Geometry check sheet. Reference: the model listing, model coordinates, mm. Give positions to 0.01 mm unless a question says otherwise; leave off trailing zeros. Loops run counter-clockwise (first coordinate to the right, second up) from the corner with the lowest first, then second, coordinate; pieces in that order, holes last. Notation, with made-up numbers: (50.5, 62.5) - (83.5, 62.5) arc R12 ccw to (83.5, 85.5) - close; hole circle Ø4 at (-33.5, 39). An arc over 180 degrees is marked (long way). Use a Markdown table: item, result. Add a question column.
1. Material ranges on L1, parallel to Y at x = -18, z = 6.25; L2, parallel to Z at x = -5, y = -38; L3, parallel to X at y = 27.5, z = 7, recorded low to high.
2. Cross-section at A-A on x = -6. Enter the section's corners in (y, z), and give its area (3 significant figures).
3. Depth check by flat-ended pin: P1, Ø0.8, axis at y = 30.5, z = 9.5, coming from the +X side; P2, Ø1.6, axis at x = -41, y = 10, coming from the +Z side. Enter the tip coordinate at first touch or a pass-through.
4. Cross-section at B-B on y = -40. Enter the section's corners in (x, z), and give its area (3 significant figures).
from build123d import *

# Parameters (mm, degrees)
F1_DEPTH = 132
F4_T     = -2


with BuildPart() as f1:
    # F0 (on Front) → F1 (new body)
    with BuildSketch(Plane.XZ):
        Polygon((-39.8409090909, -5.0908953616), (27.1590909091, -5.0908953616), (30.1590909091, -5.0908953616), (30.1590909091, -0.0908953616), (29.1590909091, 0.9091046384), (27.1590909091, 0.9091046384), (27.1590909091, 1.9091046384), (-39.8410601137, 1.909104627), (-39.8409090909, 0.9091046384), (-41.8409090909, 0.9088025928), (-42.8409090909, -0.0908953616), (-42.8409090909, -5.0908953616), align=None)
    extrude(amount=F1_DEPTH)


with BuildPart() as f1_1:
    # F2: moved
    add(f1.part.moved(Location((0, 0, 8))))


with BuildPart() as f1_2:
    # F3: moved
    add(f1_1.part.moved(Location((0, 70, 0))))

    # F4 (hollow: no face is removed)
    offset(amount=F4_T, kind=Kind.INTERSECTION, mode=Mode.SUBTRACT)


solid = f1_2.part
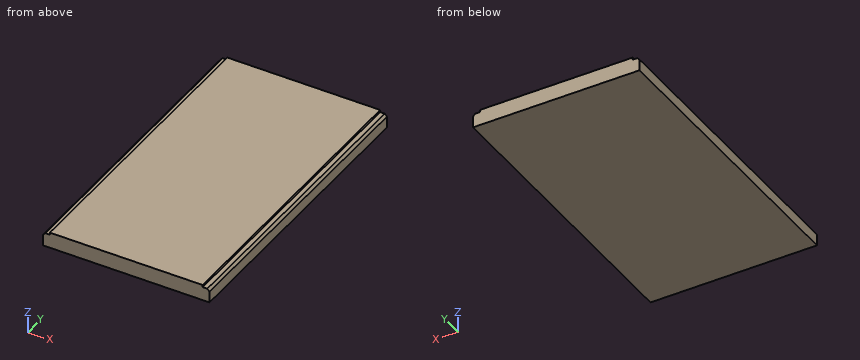
Values found:
| question | item | result |
|---|---|---|
| 1 | L1 | y = -62 to -60, 68 to 70 |
| 1 | L2 | z = 2.91 to 4.91, 7.91 to 9.91 |
| 1 | L3 | x = -42.84 to -37.84, 25.16 to 30.16 |
| 2 | outline | (-62, 2.91) - (70, 2.91) - (70, 9.91) - (-62, 9.91) - close; hole (-60, 4.91) - (68, 4.91) - (68, 7.91) - (-60, 7.91) - close |
| 2 | area | 540 mm2 |
| 3 | P1 | stops at x = 27.16 |
| 3 | P2 | stops at z = 8.91 |
| 4 | outline | (-42.84, 2.91) - (30.16, 2.91) - (30.16, 7.91) - (29.16, 8.91) - (27.16, 8.91) - (27.16, 9.91) - (-39.84, 9.91) - (-39.84, 8.91) - (-41.84, 8.91) - (-42.84, 7.91) - close; hole (-40.84, 4.91) - (28.16, 4.91) - (28.16, 6.91) - (25.16, 6.91) - (25.16, 7.91) - (-37.84, 7.91) - (-37.84, 6.91) - (-40.84, 6.91) - close |
| 4 | area | 303 mm2 |
